The model under review builds one solid part; all positions refer to its coordinate system, in mm. Face numbers are marked on the shaded views. A direction names the side the tool comes from. Round coordinates to 2 decimals unless told otherwise and drop trailing zeros. Loops run counter-clockwise (first coordinate to the right, second up) from the corner with the lowest first, then second, coordinate; pieces in that order, holes last. Notation, with made-up numbers: M 64.5,42 L 82.5,42 A21 ccw 82.5,58 Z; hole C 77,70.5 d4. An arc over 180 degrees is marked long. Use a Markdown table: item, result. Add a question column.
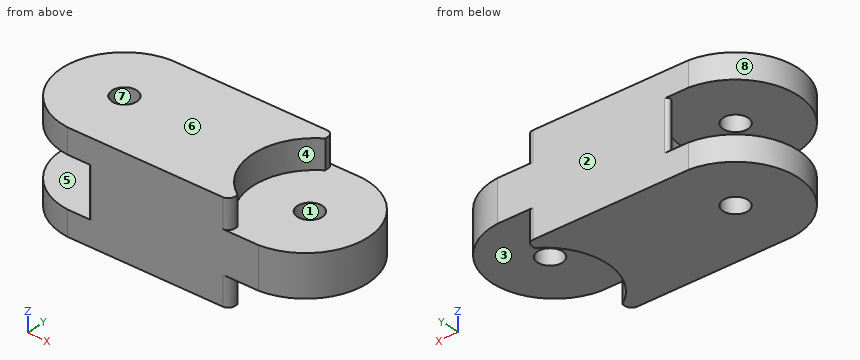
```python
from build123d import *

# Parameters (mm, degrees)
SKETCH1_W               = 29.21
SKETCH1_H               = 15.24
BOSS_EXTRUDE1_DEPTH     = 19.05
BOSS_EXTRUDE2_DEPTH     = 3.175
BOSS_EXTRUDE3_DEPTH     = 3.81
LPATTERN1_COUNT         = 2
LPATTERN1_PITCH         = 11.43
SKETCH7_R               = 1.905
CUT_EXTRUDE2_DEPTH      = 8.62
CUT_EXTRUDE2_DEPTH_BACK = 8.62
CUT_EXTRUDE4_DEPTH      = 2.794
CUT_EXTRUDE4_DEPTH_BACK = 3.175
CUT_EXTRUDE5_DEPTH      = 5.842
CUT_EXTRUDE6_DEPTH      = 3.81
FILLET2_R               = 0.5
SKETCH16_R              = 1.905
CUT_EXTRUDE8_DEPTH      = 2.27
CUT_EXTRUDE8_DEPTH_BACK = 14.97
SKETCH17_W              = 4.445
SKETCH17_H              = 4.445
CUT_EXTRUDE9_DEPTH      = 19.05
LPATTERN2_COUNT         = 2
LPATTERN2_PITCH         = 10.795
FILLET4_R               = 1


with BuildPart() as part:
    # Sketch1 → Boss-Extrude1 (new body)
    with BuildSketch(Plane(origin=(0, 0, 0), x_dir=(1, 0, 0), z_dir=(0, 1, 0))):
        Rectangle(SKETCH1_W, SKETCH1_H)
    extrude(amount=BOSS_EXTRUDE1_DEPTH)

    # Sketch3 → Boss-Extrude2 (add, symmetric)
    with BuildSketch(Plane.XY):
        with BuildLine():
            Line((14.605, 19.05), (14.605, 0))
            ThreePointArc((14.605, 0), (23.403337922, 9.525), (14.605, 19.05))
        make_face()
    extrude(amount=BOSS_EXTRUDE2_DEPTH, both=True)

    # Sketch6 → Boss-Extrude3 (add)
    with BuildSketch(Plane.XY.offset(7.62)):
        with BuildLine():
            Line((-14.605, 19.05), (-14.605, 0))
            ThreePointArc((-14.605, 0), (-23.403337922, 9.525), (-14.605, 19.05))
        make_face()
    boss_extrude3 = extrude(amount=-BOSS_EXTRUDE3_DEPTH)

    # LPattern1: Boss-Extrude3 ×2
    with Locations(*[(0, 0, -i * LPATTERN1_PITCH) for i in range(1, LPATTERN1_COUNT)]):
        add(boss_extrude3)

    # Sketch7 → Cut-Extrude2 (cut, two sides)
    with BuildSketch(Plane.XY) as cut_extrude2_sk:
        with Locations((-13.848330108, 9.525)):
            Circle(SKETCH7_R)
    extrude(amount=CUT_EXTRUDE2_DEPTH, mode=Mode.SUBTRACT)
    extrude(cut_extrude2_sk.sketch, amount=-CUT_EXTRUDE2_DEPTH_BACK, mode=Mode.SUBTRACT)

    # Sketch9 → Cut-Extrude4 (cut, two sides)
    with BuildSketch(Plane.XY.offset(6.35)) as cut_extrude4_sk:
        with BuildLine():
            Line((14.605, 19.05), (14.605, 0))
            ThreePointArc((14.605, 0), (5.806662078, 9.525), (14.605, 19.05))
        make_face()
    extrude(amount=CUT_EXTRUDE4_DEPTH, mode=Mode.SUBTRACT)
    extrude(cut_extrude4_sk.sketch, amount=-CUT_EXTRUDE4_DEPTH_BACK, mode=Mode.SUBTRACT)

    # Sketch11 → Cut-Extrude5 (cut)
    with BuildSketch(Plane.XY.offset(-9.017)):
        with BuildLine():
            Line((14.605, 19.05), (14.605, 0))
            ThreePointArc((14.605, 0), (5.806662078, 9.525), (14.605, 19.05))
        make_face()
    extrude(amount=CUT_EXTRUDE5_DEPTH, mode=Mode.SUBTRACT)

    # Sketch12 → Cut-Extrude6 (cut, symmetric)
    with BuildSketch(Plane.XY):
        with BuildLine():
            Line((-14.605, 19.05), (-14.605, 0))
            ThreePointArc((-14.605, 0), (-5.806662078, 9.525), (-14.605, 19.05))
        make_face()
    extrude(amount=CUT_EXTRUDE6_DEPTH, both=True, mode=Mode.SUBTRACT)

    # Fillet2
    fillet2_edges = [part.edges().sort_by_distance(p)[0] for p in [
        (-14.605, 0, 0),
        (-14.605, 19.05, 0),
    ]]
    fillet(fillet2_edges, radius=FILLET2_R)

    # Sketch16 → Cut-Extrude8 (cut, two sides)
    with BuildSketch(Plane.XY.offset(6.35)) as cut_extrude8_sk:
        with Locations(Location((14.513337922, 9.525, 0), (0, 0, 180))):  # turned: the seam where the file's is
            Circle(SKETCH16_R)
    extrude(amount=CUT_EXTRUDE8_DEPTH, mode=Mode.SUBTRACT)
    extrude(cut_extrude8_sk.sketch, amount=-CUT_EXTRUDE8_DEPTH_BACK, mode=Mode.SUBTRACT)

    # Sketch17 → Cut-Extrude9 (cut)
    with BuildSketch(Plane(origin=(0, 19.05, 0), x_dir=(1, 0, 0), z_dir=(0, 1, 0))):
        with Locations((12.3825, 5.3975)):
            Rectangle(SKETCH17_W, SKETCH17_H)
    cut_extrude9 = extrude(amount=-CUT_EXTRUDE9_DEPTH, mode=Mode.SUBTRACT)

    # LPattern2: Cut-Extrude9 ×2
    with Locations(*[(0, 0, i * LPATTERN2_PITCH) for i in range(1, LPATTERN2_COUNT)]):
        add(cut_extrude9, mode=Mode.SUBTRACT)

    # Fillet4
    fillet4_edges = [part.edges().sort_by_distance(p)[0] for p in [
        (10.16, 19.05, -5.3975),
        (10.16, 0, -5.3975),
        (10.16, 0, 5.3975),
        (10.16, 19.05, 5.3975),
    ]]
    fillet(fillet4_edges, radius=FILLET4_R)


solid = part.part
```
(1) Draft analysis for pull direction X (two halves, no side actions). For the marked faces 6, 7 and 8, state which applies: released by +X, released by -X, zero draft, split by the parting line, or undercut.
(2) Insertion check: pin 1 Ø6 at (y, z) = (17, -2) entering from +X; pin 2 Ø0.6 at (y, z) = (17.5, 5) entering from +X; pin 3 Ø3.5 at (x, y) = (-13.85, 9.52) entering from +Z; pin 4 Ø6 at (y, z) = (11.5, -1) entering from -X. Each pin has a flat end and moves straight along its axis. Give the tip position at first contact, or say it passes through.
(3) For the marked faces 1, 2, 3, 4 and 5, list the 3-axis set-ups (+Z, -Z, +X, -X, +Y, -Y) from which the entire face can be reached by the end or side of a thin tool; tool diameter is ignored.
(4) Consider section B-B, the plane z = -5.5. Give the boundary of the cut face in (x, y) (3 decimals).
(5) Consider section D-D, the plane x = 8. Give the boundary of the cut face in (y, z) (3 decimals).
(6) Consider section A-A, the plane x = -10. Give the boundary of the cut face in (y, z).
(7) Consider section C-C, the plane y = 4.25. Give the boundary of the cut face in (x, z) (3 decimals).
(8) To check wall thickness, follow probe 1 along Z at (x, y) = (-7.5, 13); probe 2 along Z at (x, y) = (7.5, 11) (3 decimals); probe 3 along Y at (x, z) = (-8, -3.75). State the ranges of each line that lie inside material, in increasing order.
Found:
| question | item | result |
|---|---|---|
| 1 | face 6 | zero draft |
| 1 | face 7 | undercut |
| 1 | face 8 | released by -X |
| 2 | pin 1 | stops at x = 22.29 |
| 2 | pin 2 | stops at x = 10.16 |
| 2 | pin 3 | passes through |
| 2 | pin 4 | stops at x = -23.36 |
| 3 | face 1 | +Z, -Z |
| 3 | face 2 | +Z, -Z, +X, -X, +Y |
| 3 | face 3 | -Z, +X |
| 3 | face 4 | +Z, +X |
| 3 | face 5 | -X |
| 4 | outline | M -14.605,0 L 9.16,0 A1 ccw 10.16,1 L 10.16,1.51 A9.555 cw 10.16,17.54 L 10.16,18.05 A1 ccw 9.16,19.05 L -14.605,19.05 A9.555 ccw Z; hole C -13.848,9.525 d3.81 |
| 5 | outline | M 0,-7.62 L 3.434,-7.62 L 3.434,-3.175 L 15.616,-3.175 L 15.616,-7.62 L 19.05,-7.62 L 19.05,7.62 L 15.616,7.62 L 15.616,3.175 L 3.434,3.175 L 3.434,7.62 L 0,7.62 Z |
| 6 | outline | M 0,-7.62 L 19.05,-7.62 L 19.05,7.62 L 0,7.62 Z; hole M 1.62,-3.81 L 17.43,-3.81 L 17.43,3.81 L 1.62,3.81 Z |
| 7 | outline | M -21.815,-7.62 L 7.395,-7.62 L 7.395,-3.175 L 21.815,-3.175 L 21.815,3.175 L 7.395,3.175 L 7.395,7.62 L -21.815,7.62 L -21.815,3.81 L -7.395,3.81 L -7.395,-3.81 L -21.815,-3.81 Z |
| 8 | probe 1 | z = -7.62 to -3.81, 3.81 to 7.62 |
| 8 | probe 2 | z = -3.175 to 3.175 |
| 8 | probe 3 | y = 0 to 3.43, 15.62 to 19.05 |
